Read the model definition and answer for the solid it produces. Units are mm, in the model's axes. A direction names the side the tool comes from. Round coordinates to 2 decimals unless told otherwise and drop trailing zeros. Order: outer loops, then holes, each group sorted by start corner. A loop starts at its lowest first (then second) coordinate and runs counter-clockwise, first axis right, second up.
from build123d import *

# Parameters (mm, degrees)
SKETCH2_W               = 2
SKETCH2_H               = 3
CUT_EXTRUDE1_DEPTH      = 6
CUT_EXTRUDE1_DEPTH_BACK = 6


with BuildPart() as part:
    # Sketch1 → Revolve1 (revolve)
    with BuildSketch(Plane.XY):
        with BuildLine():
            Line((0, 12.68337521), (0, 0))
            Line((0, 0), (2, 0))
            Line((2, 0), (2, 1))
            Line((2, 1), (3, 1))
            Line((3, 1), (3, 8))
            Line((3, 8), (5, 8))
            Line((5, 8), (5, 10))
            ThreePointArc((5, 10), (2.837274331, 11.970139283), (0, 12.68337521))
        make_face()
    revolve(axis=Axis((0, 15.248921205, 0), (0, -1, 0)))

    # Sketch2 → Cut-Extrude1 (cut, two sides)
    with BuildSketch(Plane.XY) as cut_extrude1_sk:
        with Locations((0, 12.18337521)):
            Rectangle(SKETCH2_W, SKETCH2_H)
    extrude(amount=CUT_EXTRUDE1_DEPTH, mode=Mode.SUBTRACT)
    extrude(cut_extrude1_sk.sketch, amount=-CUT_EXTRUDE1_DEPTH_BACK, mode=Mode.SUBTRACT)


solid = part.part
Q1. A cutting plane is placed at A-A, the plane x = 0. Give the vertices of the cut face in (y, z).
Outcome:
outline: (0, -2) - (1, -2) - (1, -3) - (8, -3) - (8, -5) - (10, -5) arc R6 ccw to (10.68, -4.47) - (10.68, 4.47) arc R6 ccw to (10, 5) - (8, 5) - (8, 3) - (1, 3) - (1, 2) - (0, 2) - close
Q2. For faces 5 (the face through (-1.08, 9.01, -4.88)), 6 (the face through (-0.434, 0.507, -1.952)), 7 (the face through (0, 10.683, 0)), determine the directions among +Z, -Z, +X, -X, +Y, -Y from which every point of the face is accessible in a straight line to the end or side of a thin tool.
Outcome:
face 5: +Y, -Y
face 6: -Y
face 7: +Z, -Z, +Y
Q3. Straight lines are drawn through the part: probe 1 along Y at (x, z) = (0, -4); probe 2 along Y at (x, z) = (0.25, 1.5); probe 3 along Z at (x, y) = (4, 9.75). For each, find the intervals that lie inside material, in ascending order.
Outcome:
probe 1: y = 8 to 10.68
probe 2: y = 0 to 10.68
probe 3: z = -3 to 3
Q4. A cutting plane is placed at D-D, the plane x = -1.75. Give the vertices of the cut face in (y, z), plus the area to 3 significant figures.
Outcome:
outline: (0, -0.97) - (1, -0.97) - (1, -2.44) - (8, -2.44) - (8, -4.68) - (10, -4.68) arc R5.74 ccw to (10, 4.68) - (8, 4.68) - (8, 2.44) - (1, 2.44) - (1, 0.97) - (0, 0.97) - close
area: 70.7 mm2
Q5. For a pull along X with two mould halves and no side action, classify faces 1 (the face through (-1, 11, 0)), 2 (the face through (-3, 5, 0)), 3 (the face through (1, 11, 0)), 4 (the face through (0, 0, 0)) as released by +X, released by -X, zero draft, split by the parting line, or undercut.
Outcome:
face 1: undercut
face 2: split by the parting line
face 3: undercut
face 4: zero draft
Q6. A cutting plane is placed at C-C, the plane y = 4. Give the vertices of the cut face in (x, z).
Outcome:
outline: circle Ø6 at (0, 0)
Q7. Flat-ended cylindrical pins translate along their axes: pin 1 (1 mm diameter, centred on y = 11.5, z = -1.5, fed in from -X); pin 2 (1 mm diameter, centred on y = 2, z = 2, fed in from -X); pin 3 (2 mm diameter, centred on y = 11.5, z = -1, fed in from +X). Find the tip coordinate at first contact, or state that the pin passes through.
Outcome:
pin 1: stops at x = -3.92
pin 2: stops at x = -2.6
pin 3: stops at x = 4.54
Q8. A cutting plane is placed at B-B, the plane z = 0. Give the vertices of the cut face in (x, y).
Outcome:
outline: (-5, 8) - (-3, 8) - (-3, 1) - (-2, 1) - (-2, 0) - (2, 0) - (2, 1) - (3, 1) - (3, 8) - (5, 8) - (5, 10) arc R6 ccw to (1, 12.6) - (1, 10.68) - (-1, 10.68) - (-1, 12.6) arc R6 ccw to (-5, 10) - close
